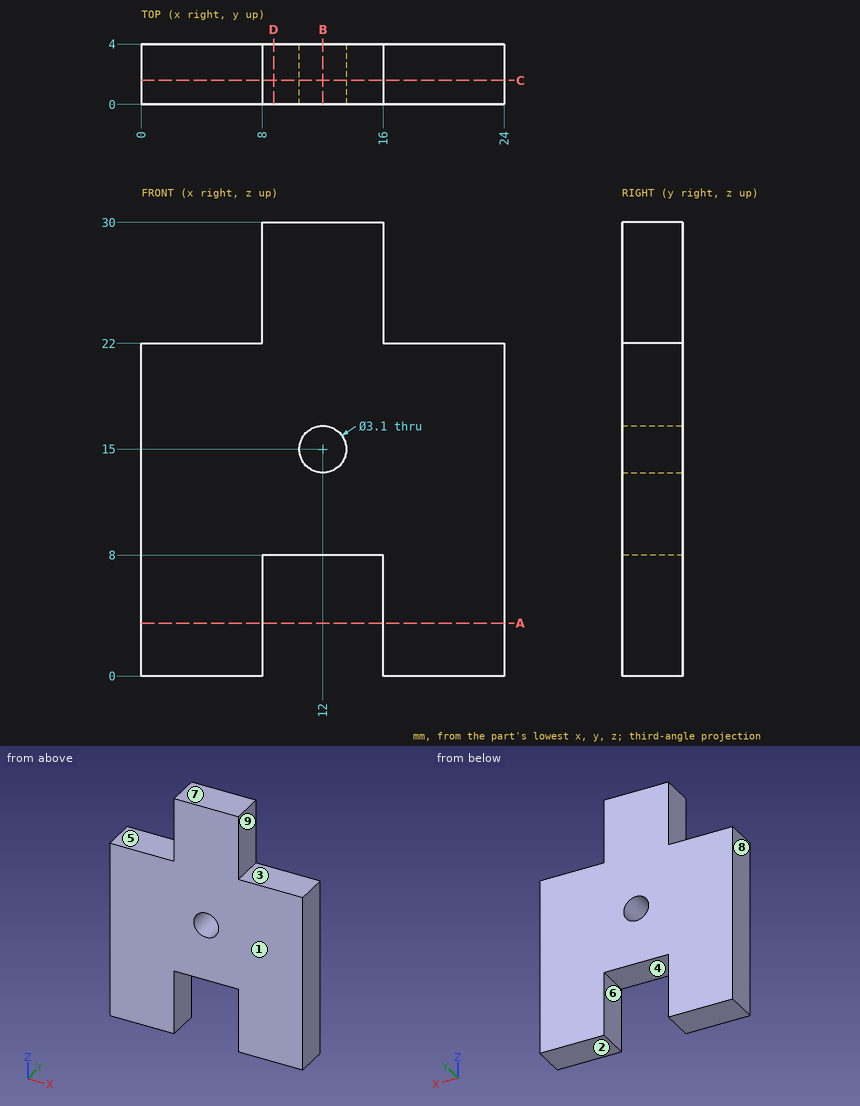
Geometry: see drawing. Coordinates: mm, zero at the bounding-box minimum. A direction names the side the tool comes from. Give positions to 0.01 mm unless a question says otherwise; leave off trailing zeros. Write each loop counter-clockwise with the first axis right and the second up, starting at its lowest first coordinate (ties: lowest second). Pieces come first, ordered by that corner, then holes. Notation, with made-up numbers: M 36.25,54 L 43.25,54 A15 cw 43.25,69 Z; hole C 61,49 d3. An arc over 180 degrees is marked long. Return JSON: item names as keys, results as strings. Group by question number.
1) Cut plane D-D, the plane x = 8.75. Output: boundary loops of the cut face in (y, z).
2) Cut plane B-B, the plane x = 12. Output: boundary loops of the cut face in (y, z), then the cut area to 3 significant figures.
3) Cut plane A-A, the plane z = 3.5. Output: boundary loops of the cut face in (x, y), then the cut area to 3 significant figures.
4) Ray query, L1, parallel to X at y = 2.75, z = 15; L2, parallel to Z at x = 12, y = 1.1; L3, parallel to Z at x = 19.25, y = 1.75. Return the intervals inside material, ascending.
5) Cut plane C-C, the plane y = 1.6. Output: boundary loops of the cut face in (x, z), then the cut area to 3 significant figures.
6) Set-up query: the marked faces 1, 2, 3, 4 and 5. Return all of +Z, -Z, +X, -X, +Y, -Y with unobstructed straight access to the full face (end or side cutting, diameter ignored); none if empty.
7) First-contact query: pin 1 Ø1.2 at (x, y) = (19, 2.5) entering from +Z; pin 2 Ø3 at (x, z) = (12, 15) entering from -Y; pin 3 Ø2 at (x, y) = (2.5, 3) entering from -Z; pin 4 Ø1.2 at (x, y) = (12, 2.5) entering from -Z. Flat tips, straight axial feed; report the tip coordinate or a pass-through.
8) Draft query along X for the marked faces 6, 7, 8 and 9. Return one class per face: released by +X, released by -X, zero draft, split by the parting line, or undercut.
Data:
{
 "1": {"outline": "M 0,8 L 4,8 L 4,30 L 0,30 Z"},
 "2": {"outline": "M 0,8 L 4,8 L 4,13.45 L 0,13.45 Z; M 0,16.55 L 4,16.55 L 4,30 L 0,30 Z", "area": "75.6 mm²"},
 "3": {"outline": "M 0,0 L 8,0 L 8,4 L 0,4 Z; M 16,0 L 24,0 L 24,4 L 16,4 Z", "area": "64.0 mm²"},
 "4": {"L1": "x = 0 to 10.45, 13.55 to 24", "L2": "z = 8 to 13.45, 16.55 to 30", "L3": "z = 0 to 22"},
 "5": {"outline": "M 0,0 L 8,0 L 8,8 L 16,8 L 16,0 L 24,0 L 24,22 L 16,22 L 16,30 L 8,30 L 8,22 L 0,22 Z; hole C 12,15 d3.1", "area": "520 mm²"},
 "6": {"face 1": "+Z, -Z, +X, -X, -Y", "face 2": "-Z, +X, -X, +Y, -Y", "face 3": "+Z, +X, +Y, -Y", "face 4": "-Z, +Y, -Y", "face 5": "+Z, -X, +Y, -Y"},
 "7": {"pin 1": "stops at z = 22", "pin 2": "passes through", "pin 3": "stops at z = 0", "pin 4": "stops at z = 8"},
 "8": {"face 6": "undercut", "face 7": "zero draft", "face 8": "released by -X", "face 9": "released by +X"}
}
